Can you work these out from the model? Positions are in its coordinate system, mm. A direction names the side the tool comes from. Give positions to 0.01 mm unless a question says otherwise; leave off trailing zeros. Write each loop counter-clockwise with the first axis right and the second up, starting at its lowest first coordinate (ties: lowest second). Pieces come first, ordered by that corner, then holes. Notation, with made-up numbers: (9.25, 59) -> (51.25, 59) arc R26 cw to (51.25, 79) -> close; hole circle Ø8 at (63.5, 85). An arc over 180 degrees is marked (long way). One line per item, written item: value.
from build123d import *

# Parameters (mm, degrees)
F0_W      = 115
F0_H      = 140
F1_DEPTH  = 2
F2_W      = 115
F2_H      = 140
F2_W_2    = 111
F2_H_2    = 136
F3_DEPTH  = 30
F4_W      = 119
F4_H      = 144
F4_W_2    = 115
F4_H_2    = 140
F5_DEPTH  = 18
F6_W      = 19
F6_H      = 3.2217571437
F6_H_2    = 32
F7_DEPTH  = 5
F8_W      = 20
F8_H      = 11
F9_DEPTH  = 2
F10_R     = 5
F11_R     = 3
F12_R     = 2
F13_R     = 1.4
F14_DEPTH = 117.001


with BuildPart() as f1:
    # F0 (on Top) → F1 (new body)
    with BuildSketch(Plane.XY):
        Rectangle(F0_W, F0_H)
    extrude(amount=F1_DEPTH)

    # F2 (on face) → F3 (join)
    with BuildSketch(Plane.XY.offset(2)):
        Rectangle(F2_W, F2_H)
        Rectangle(F2_W_2, F2_H_2, mode=Mode.SUBTRACT)
    extrude(amount=F3_DEPTH)

    # F4 (on Top) → F5 (join)
    with BuildSketch(Plane.XY):
        Rectangle(F4_W, F4_H)
        Rectangle(F4_W_2, F4_H_2, mode=Mode.SUBTRACT)
    extrude(amount=F5_DEPTH)

    # F6 (on face) → F7 (cut, symmetric)
    with BuildSketch(Plane(origin=(0, -68, 0), x_dir=(-1, 0, 0), z_dir=(0, 1, 0))):
        with Locations((18, 43.6108785719)):
            Rectangle(F6_W, F6_H)
        with Locations((18, 26)):
            Rectangle(F6_W, F6_H_2)
        with BuildLine():
            Line((-17, 10), (-6, 10))
            Line((-6, 10), (-6, 23))
            ThreePointArc((-6, 23), (-11.5, 25.6698729811), (-17, 23))
            Line((-17, 23), (-17, 10))
        make_face()
    extrude(amount=F7_DEPTH, both=True, mode=Mode.SUBTRACT)

    # F8 (on face) → F9 (cut)
    with BuildSketch(Plane(origin=(0, 70, 0), x_dir=(-1, 0, 0), z_dir=(0, 1, 0))):
        with Locations((28, 33.5)):
            Rectangle(F8_W, F8_H)
    extrude(amount=-F9_DEPTH, mode=Mode.SUBTRACT)

    # F10
    f10_edges = [f1.edges().sort_by_distance(p)[0] for p in [
        (-59.5, -72, 9),
        (59.5, -72, 9),
        (-59.5, 72, 9),
        (59.5, 72, 9),
    ]]
    fillet(f10_edges, radius=F10_R)

    # F11
    f11_edges = [f1.edges().sort_by_distance(p)[0] for p in [
        (-57.5, -70, 25),
        (57.5, -70, 25),
        (57.5, 70, 25),
        (-57.5, 70, 25),
    ]]
    fillet(f11_edges, radius=F11_R)

    # F12
    f12_edges = [f1.edges().sort_by_distance(p)[0] for p in [
        (-55.5, -68, 17),
        (55.5, -68, 17),
        (55.5, 68, 17),
        (-55.5, 68, 17),
    ]]
    fillet(f12_edges, radius=F12_R)

    # F13 (on face) → F14 (cut, through all)
    with BuildSketch(Plane(origin=(-57.5, 0, 0), x_dir=(0, -1, 0), z_dir=(-1, 0, 0))):
        with Locations((-37, 25)):
            Circle(F13_R)
        with Locations((37, 25)):
            Circle(F13_R)
    extrude(amount=-F14_DEPTH, mode=Mode.SUBTRACT)


solid = f1.part
1) Will these pins go through, and if not, where does the flat tip stop? pin 1 (1.6 mm diameter, centred on y = 69, z = 31, fed in from -X); pin 2 (7 mm diameter, centred on x = -42, z = 28, fed in from -Y); pin 3 (4 mm diameter, centred on y = -1.5, z = 23, fed in from +X).
Answer list:
pin 1: stops at x = -57.25
pin 2: stops at y = -70
pin 3: stops at x = 57.5
2) If we section it at C-C (y = 41): Write out the boundary of the cut face in (x, z).
Answer list:
outline: (-59.5, 0) -> (59.5, 0) -> (59.5, 18) -> (57.5, 18) -> (57.5, 32) -> (55.5, 32) -> (55.5, 2) -> (-55.5, 2) -> (-55.5, 32) -> (-57.5, 32) -> (-57.5, 18) -> (-59.5, 18) -> close
3) I need wall thicknesses on L1, parallel to Y at x = -44, z = 9.5; L2, parallel to Y at x = 45, z = 27; L3, parallel to X at y = -37.5, z = 8. Which ranges of each line are inside material? Lowest first, please.
Answer list:
L1: y = -72 to -68, 68 to 72
L2: y = -70 to -68, 68 to 70
L3: x = -59.5 to -55.5, 55.5 to 59.5
4) If we section it at A-A (z = 8): Write out the boundary of the cut face in (x, y), and give its area (3 significant figures).
Answer list:
outline: (-59.5, -67) arc R5 ccw to (-54.5, -72) -> (54.5, -72) arc R5 ccw to (59.5, -67) -> (59.5, 67) arc R5 ccw to (54.5, 72) -> (-54.5, 72) arc R5 ccw to (-59.5, 67) -> close; hole (-55.5, -66) arc R2 ccw to (-53.5, -68) -> (53.5, -68) arc R2 ccw to (55.5, -66) -> (55.5, 66) arc R2 ccw to (53.5, 68) -> (-53.5, 68) arc R2 ccw to (-55.5, 66) -> close
area: 2,020 mm^2
5) If we section it at B-B (x = 45.5): Write out the boundary of the cut face in (y, z), and give its area (3 significant figures).
Answer list:
outline: (-72, 0) -> (72, 0) -> (72, 18) -> (70, 18) -> (70, 32) -> (68, 32) -> (68, 2) -> (-68, 2) -> (-68, 32) -> (-70, 32) -> (-70, 18) -> (-72, 18) -> close
area: 472 mm^2
6) We'd pull the mould along Y, two halves only. Please class faces 6 (the face through (-56.64, 69.1, 24.9)), 7 (the face through (-57.5, -1, 25)), 8 (the face through (-1, 68, 17)): released by +Y, released by -Y, zero draft, split by the parting line, or undercut.
Answer list:
face 6: released by +Y
face 7: zero draft
face 8: undercut
7) For faces 1 (the face through (23, -70, 25)), 2 (the face through (17, -70, 15)), 3 (the face through (56.6, 69.14, 24.9)), 4 (the face through (-1, 70, 25)), 5 (the face through (-18, -70, 10)), which set-ups out of +Z, -Z, +X, -X, +Y, -Y let a thin tool reach every point of the face, with its end or its side?
Answer list:
face 1: +Z, +X, -X, -Y
face 2: -Y
face 3: +Z, +X, +Y
face 4: +Z, +X, -X, +Y
face 5: +Z, -Y
